```python
from build123d import *

# Parameters (mm, degrees)
EXTRUDE_START      = 300
EXTRUDE_SKETCH_1_R = 15
EXTRUDE_1_DEPTH    = 18
EXTRUDE_START_2    = 318
EXTRUDE_SKETCH_2_R = 9
EXTRUDE_2_DEPTH    = 237


with BuildPart() as part:
    # Extrude sketch 1 → Extrude 1 (new body)
    with BuildSketch(Plane.XY.offset(EXTRUDE_START)):
        with Locations((860, -225)):
            Circle(EXTRUDE_SKETCH_1_R)
    extrude(amount=EXTRUDE_1_DEPTH)


with BuildPart() as body_2:
    # Extrude sketch 2 → Extrude 2 (new body)
    with BuildSketch(Plane.XY.offset(EXTRUDE_START_2)):
        with Locations((860, -225)):
            Circle(EXTRUDE_SKETCH_2_R)
    extrude(amount=EXTRUDE_2_DEPTH)


with BuildPart() as body_3:
    # Revolve profile 1 → Revolve 1 (revolve)
    with BuildSketch(Plane(origin=(0, -225, 0), x_dir=(1, 0, 0), z_dir=(0, 1, 0)), mode=Mode.PRIVATE) as revolve_1_sk:
        Polygon((860, -555), (869, -555), (866, -561), (860, -563), align=None)
    revolve(revolve_1_sk.sketch.rotate(Axis((860, -225, 550), (0, 0, 1)), 180), axis=Axis((860, -225, 550), (0, 0, 1)))


with BuildPart() as part_1:
    add(part.part)

    # Combine _weld _ assembly of features: union body 2, body 3
    add(body_2.part)
    add(body_3.part)


solid = part_1.part
```
Build history of the part. All positions in model axes, mm. A direction names the side the tool comes from. Round coordinates to 2 decimals unless told otherwise and drop trailing zeros. Write each loop counter-clockwise with the first axis right and the second up, starting at its lowest first coordinate (ties: lowest second). Pieces come first, ordered by that corner, then holes. Notation, with made-up numbers: (77, 9) - (127, 9) arc R8 ccw to (127, 21) - close; hole circle Ø8 at (-24, 47.25). An arc over 180 degrees is marked (long way). Write each question's results on one line, items separated by ' | '. Start each with the question number.
Item 1: Which spindle directions (+Z, -Z, +X, -X, +Y, -Y) get a long thin tool onto all of the face, cutting with end or side? Do faces 1 (the face through (858.828, -216.077, 434.841)), 2 (the face through (873.856, -230.745, 308.874)). Say none if no direction does.
Item 2: Wall check: L1, parallel to Z at x = 853, y = -216.5; L2, parallel to X at y = -228.5, z = 545.5; L3, parallel to Z at x = 863.5, y = -226.5. Give the ranges that are in metal, low to high. Write a range as [from, to].
Item 3: Drop flat-ended pins along their axis: P1, Ø6, axis at x = 854, z = 395, coming from the +Y side; P2, Ø6, axis at y = -226.5, z = 361, coming from the -X side; P3, Ø1.5, axis at x = 857, z = 408.5, coming from the -Y side; P4, Ø12, axis at x = 859, y = -229, coming from the +Z side. Give the stop position or say it passes through.
Item 4: Saw through at A-A (z = 472.5). Write the cut outline in (x, y).
Results are:
1) face 1: +Z | face 2: +Z, -Z
2) L1: z = [300, 318] | L2: x = [851.71, 868.29] | L3: z = [300, 561.73]
3) P1: stops at y = -216.51 | P2: stops at x = 851 | P3: stops at y = -233.71 | P4: stops at z = 563
4) outline: circle Ø18 at (860, -225)
